from build123d import *

# Parameters (mm, degrees)
F0_W     = 32
F0_H     = 32
F1_DEPTH = 1.6
F2_W     = 25
F2_H     = 18
F3_DEPTH = 10
F4_R     = 7.5
F5_DEPTH = 10
F6_W     = 4
F6_H     = 10.84
F6_H_2   = 6
F7_DEPTH = 5
F8_R     = 1.25
F9_DEPTH = 25


with BuildPart() as f1:
    # F0 (on Front) → F1 (new body)
    with BuildSketch(Plane.XZ):
        Rectangle(F0_W, F0_H)
    extrude(amount=F1_DEPTH)

    # F2 (on face) → F3 (join)
    with BuildSketch(Plane.XZ.offset(1.6)):
        Rectangle(F2_W, F2_H)
    extrude(amount=F3_DEPTH)

    # F4 (on face) → F5 (join)
    with BuildSketch(Plane.XZ.offset(11.6)):
        Circle(F4_R)
    extrude(amount=F5_DEPTH)

    # F6 (on face) → F7 (join)
    with BuildSketch(Plane(origin=(0, 0, 0), x_dir=(-1, 0, 0), z_dir=(0, 1, 0))):
        with Locations((14, 6.7)):
            Rectangle(F6_W, F6_H)
        with Locations((14, -8.5)):
            Rectangle(F6_W, F6_H_2)
    extrude(amount=F7_DEPTH)

    # F8 (on face) → F9 (cut)
    with BuildSketch(Plane.XZ.offset(1.6)):
        with Locations((14, 14)):
            Circle(F8_R)
        with Locations((14, -14)):
            Circle(F8_R)
        with Locations((-14, -14)):
            Circle(F8_R)
        with Locations((-14, 14)):
            Circle(F8_R)
    extrude(amount=-F9_DEPTH, mode=Mode.SUBTRACT)


solid = f1.part
Source: CAD feature listing. Evaluate the final solid. Frame: model axes, mm. A direction names the side the tool comes from. Give positions to 0.01 mm unless a question says otherwise; leave off trailing zeros. Write each loop counter-clockwise with the first axis right and the second up, starting at its lowest first coordinate (ties: lowest second). Pieces come first, ordered by that corner, then holes. Notation, with made-up numbers: (76, -1) -> (128, -1) arc R18 ccw to (128, 17) -> close; hole circle Ø6 at (88, 18.5). An arc over 180 degrees is marked (long way). Return JSON: item names as keys, results as strings. Group by question number.
1. Section C-C, the plane x = 0. Output: boundary loops of the cut face in (y, z), then the cut area to 3 significant figures.
2. Section B-B, the plane z = 0. Output: boundary loops of the cut face in (x, y).
3. Section D-D, the plane y = -17.5. Output: boundary loops of the cut face in (x, z).
4. Pin query (flat end, axial travel): pin 1 Ø4 at (y, z) = (-5, 4) entering from +X; pin 2 Ø5 at (x, z) = (8.5, 12.5) entering from -Y; pin 3 Ø5 at (x, y) = (1.5, -5) entering from -Z; pin 4 Ø2 at (x, z) = (-14, -14) entering from +Y. Return the tip coordinate at first contact, or that it passes through.
5. Material intervals for line 1 (Z direction, x = 14, y = -0.5); line 2 (Y direction, x = -2.5, z = -9.5); line 3 (X direction, y = -2.75, z = -2), sorted ascending. Write a range as from..to.
6. Section A-A, the plane x = 14. Output: boundary loops of the cut face in (y, z), then the cut area to 3 significant figures.
7. Access query for faces 1 (the face through (0, -7, 9)), 2 (the face through (0, -11.6, -8)), 3 (the face through (-12.5, -7, 0)). Directions: +Z, -Z, +X, -X, +Y, -Y. A direction counts if a zero-diameter tool reaches every point of the face in a straight line with its end or side. Return the directions, or none.
Determined:
{
 "1": {"outline": "(-21.6, -7.5) -> (-11.6, -7.5) -> (-11.6, -9) -> (-1.6, -9) -> (-1.6, -16) -> (0, -16) -> (0, 16) -> (-1.6, 16) -> (-1.6, 9) -> (-11.6, 9) -> (-11.6, 7.5) -> (-21.6, 7.5) -> close", "area": "381 mm2"},
 "2": {"outline": "(-16, -1.6) -> (-12.5, -1.6) -> (-12.5, -11.6) -> (-7.5, -11.6) -> (-7.5, -21.6) -> (7.5, -21.6) -> (7.5, -11.6) -> (12.5, -11.6) -> (12.5, -1.6) -> (16, -1.6) -> (16, 0) -> (-16, 0) -> close"},
 "3": {"outline": "circle Ø15 at (0, 0)"},
 "4": {"pin 1": "stops at x = 12.5", "pin 2": "stops at y = -1.6", "pin 3": "stops at z = -9", "pin 4": "passes through"},
 "5": {"line 1": "z = -16..-15.25, -12.75..12.75, 15.25..16", "line 2": "y = -1.6..0", "line 3": "x = -12.5..12.5"},
 "6": {"outline": "(-1.6, -16) -> (0, -16) -> (0, -15.25) -> (-1.6, -15.25) -> close; (-1.6, -12.75) -> (0, -12.75) -> (0, 12.75) -> (-1.6, 12.75) -> close; (-1.6, 15.25) -> (0, 15.25) -> (0, 16) -> (-1.6, 16) -> close", "area": "43.2 mm2"},
 "7": {"face 1": "+Z, +X, -X, -Y", "face 2": "-Y", "face 3": "+Z, -Z, -X, -Y"}
}
